```python
from build123d import *

# Parameters (mm, degrees)
SKETCH1_R           = 1.5
BOSS_EXTRUDE1_DEPTH = 3.9
BOSS_EXTRUDE2_START = 2.1
SKETCH1_3_R         = 7.45
SKETCH1_3_R_2       = 1.5
BOSS_EXTRUDE2_DEPTH = 2.1
FILLET1_R           = 10


with BuildPart() as part:
    # Sketch1 → Boss-Extrude1 (new body)
    with BuildSketch(Plane(origin=(0, 0, 0), x_dir=(1, 0, 0), z_dir=(0, 1, 0))):
        with BuildLine():
            ThreePointArc((6.451889258, 3.725), (-7.45, 0), (6.451889258, -3.725))
            Line((6.451889258, -3.725), (24.0716503, -3.725))
            ThreePointArc((24.0716503, -3.725), (27.7966503, 0), (24.0716503, 3.725))
            Line((24.0716503, 3.725), (6.451889258, 3.725))
        make_face()
        with Locations(Location((0, 0, 0), (0, 0, 270))):
            Circle(SKETCH1_R, mode=Mode.SUBTRACT)
        with Locations(Location((8.95, 0, 0), (0, 0, 270))):
            Circle(SKETCH1_R, mode=Mode.SUBTRACT)
        with Locations(Location((20.0716503, 0, 0), (0, 0, 270))):
            Circle(SKETCH1_R, mode=Mode.SUBTRACT)
        with Locations(Location((24.0716503, 0, 0), (0, 0, 270))):
            Circle(SKETCH1_R, mode=Mode.SUBTRACT)
    extrude(amount=-BOSS_EXTRUDE1_DEPTH)

    # Sketch1_3 → Boss-Extrude2 (add)
    # profile 1 of 2: a face of its own
    with BuildSketch(Plane(origin=(0, 0, 0), x_dir=(1, 0, 0), z_dir=(0, 1, 0)).offset(BOSS_EXTRUDE2_START)):
        with Locations(Location((0, 0, 0), (0, 0, 270))):
            Circle(SKETCH1_3_R)
        with Locations(Location((0, 0, 0), (0, 0, 270))):
            Circle(SKETCH1_3_R_2, mode=Mode.SUBTRACT)
    # profile 2 of 2: a face of its own
    with BuildSketch(Plane(origin=(0, 0, 0), x_dir=(1, 0, 0), z_dir=(0, 1, 0)).offset(BOSS_EXTRUDE2_START)):
        with BuildLine():
            Line((20.0716503, -3), (24.0716503, -3))
            ThreePointArc((24.0716503, -3), (27.0716503, 0), (24.0716503, 3))
            Line((24.0716503, 3), (20.0716503, 3))
            ThreePointArc((20.0716503, 3), (17.0716503, 0), (20.0716503, -3))
        make_face()
        with Locations(Location((20.0716503, 0, 0), (0, 0, 270))):
            Circle(SKETCH1_3_R_2, mode=Mode.SUBTRACT)
        with Locations(Location((24.0716503, 0, 0), (0, 0, 270))):
            Circle(SKETCH1_3_R_2, mode=Mode.SUBTRACT)
    extrude(amount=-BOSS_EXTRUDE2_DEPTH)

    # Fillet1
    # the kernel refuses this fillet: 10 mm, written as the material it adds along each edge
    with BuildSketch(Plane(origin=(6.451889258, 0, 3.725), x_dir=(1, 0, 0), z_dir=(0, -1, 0))) as fillet1_piece_1:
        with BuildLine():
            CenterArc((4.32432877, 10), FILLET1_R, 231.86268063, 38.13731937)
            ThreePointArc((-1.851154341, 2.134670487), (-0.823449882, 1.155898502), (0, 0))
            Line((0, 0), (4.32432877, 0))
        make_face()
    extrude(amount=3.9)
    with BuildSketch(Plane(origin=(6.451889258, 0, -3.725), x_dir=(1, 0, 0), z_dir=(0, -1, 0))) as fillet1_piece_2:
        with BuildLine():
            CenterArc((4.32432877, -10), FILLET1_R, 90, 38.13731937)
            ThreePointArc((-1.851154341, -2.134670487), (-0.823449882, -1.155898502), (0, 0))
            Line((0, 0), (4.32432877, 0))
        make_face()
    extrude(amount=3.9)


solid = part.part
```
Read the model definition and answer for the solid it produces. Units are mm, in the model's axes. A direction names the side the tool comes from. Give positions to 0.01 mm unless a question says otherwise; leave off trailing zeros. Loops run counter-clockwise (first coordinate to the right, second up) from the corner with the lowest first, then second, coordinate; pieces in that order, holes last.
Item 1: The mould has two halves that part along X. Classify faces 5 (the cylindrical face through (25.336, -0.858, 0.806)), 6 (the cylindrical face through (27.07, 1.06, 0.07)), 7 (the flat face through (7, -3.9, 0)), 8 (the flat face through (15, 0, 0)): released by +X, released by -X, zero draft, split by the parting line, or undercut.
Item 2: The part is cut by section A-A (y = 1.55). Write down the section's boundary in (x, z).
Item 3: The part is cut by section D-D (x = 15). Write down the section's boundary in (y, z) (3 decimals).
Item 4: The part is cut by section B-B (x = 0). Write down the section's boundary in (y, z), and give its area (3 significant figures).
Item 5: Each of these flat-tipped pins is pushed along its axis until it touches: pin 1 Ø1 at (x, y) = (20.5, -2.5) entering from -Z (3 decimals); pin 2 Ø1.7 at (x, y) = (21.5, 1) entering from -Z; pin 3 Ø1 at (x, y) = (21.5, 1.5) entering from +Z; pin 4 Ø1.8 at (x, z) = (0, 0) entering from +Y. Where does it stop, or does it pass through?
Item 6: For faces 1 (the flat face through (22, 1, 3)), 2 (the flat face through (22, 1, -3)), 3 (the flat face through (17, -2, 3.725)), 4 (the cylindrical face through (17.072, 1.065, -0.066)), determine the directions among +Z, -Z, +X, -X, +Y, -Y from which every point of the face is accessible in a straight line to the end or side of a thin tool.
Item 7: The part is cut by section C-C (z = -5). Write down the section's boundary in (x, y), and give its area (3 significant figures).
Item 8: Find the intervals of material crossed by line 1 along X through (y, z) = (-1.55, 0); line 2 along X through (y, z) = (0.55, 0); line 3 along Y through (x, z) = (13.5, 0), in increasing order.
Taken from the geometry:
1. face 5: undercut
1. face 6: released by +X
1. face 7: zero draft
1. face 8: undercut
2. outline: circle Ø14.9 at (0, 0); (20.07, -3) - (24.07, -3) arc R3 ccw to (24.07, 3) - (20.07, 3) arc R3 ccw to start; hole circle Ø3 at (0, 0); hole circle Ø3 at (20.07, 0); hole circle Ø3 at (24.07, 0)
3. outline: (-3.9, -3.725) - (0, -3.725) - (0, 3.725) - (-3.9, 3.725) - close
4. outline: (-3.9, -7.45) - (2.1, -7.45) - (2.1, -1.5) - (-3.9, -1.5) - close; (-3.9, 1.5) - (2.1, 1.5) - (2.1, 7.45) - (-3.9, 7.45) - close
4. area: 71.4 mm2
5. pin 1: stops at z = -3.725
5. pin 2: stops at z = -3
5. pin 3: stops at z = 3
5. pin 4: passes through
6. face 1: +Z, +X, +Y
6. face 2: -Z, +X, +Y
6. face 3: +Z, +X, +Y, -Y
6. face 4: +Y
7. outline: (-5.52, -3.9) - (5.89, -3.9) - (5.89, 0) - (5.52, 0) - (5.52, 2.1) - (-5.52, 2.1) - close
7. area: 67.7 mm2
8. line 1: x = -7.45 to -1.5, 1.5 to 7.45, 10.45 to 18.57, 21.57 to 22.57, 25.57 to 27.8
8. line 2: x = -7.45 to -1.5, 1.5 to 7.45, 17.07 to 18.57, 21.57 to 22.57, 25.57 to 27.07
8. line 3: y = -3.9 to 0
